Verification items for this drawing (mm, ordinates from the low corner). A direction names the side the tool comes from. Coordinates: 2 decimals unless noted, no trailing zeros. Order: outer loops, then holes, each group sorted by start corner. A loop starts at its lowest first (then second) coordinate and runs counter-clockwise, first axis right, second up. Notation, with made-up numbers: M -26.5,58.25 L 30.5,58.25 A18 cw 30.5,89.25 Z; hole C 48,43.25 d8. An arc over 180 degrees is marked long. Answer as a JSON object with one key per item and string values. Group by question number.
(1) Access from +Z, -Z, +X, -X, +Y, -Y to the whole of each face (thin tool, end or side, straight path). Record for the marked faces 5, 6 and 7.
(2) Material ranges on line 1 (Y direction, x = 15, z = 2.75); line 2 (X direction, y = 10, z = 8.25) (1 decimal); line 3 (X direction, y = 4.75, z = 5.5) (1 decimal), recorded low to high.
(3) Cross-section at D-D (x = 11.5). Enter the section's corners in (y, z).
(4) Cross-section at B-B (z = 6). Enter the section's corners in (x, y) (1 decimal).
(5) Cross-section at C-C (y = 13.5). Enter the section's corners in (x, z), plus the area to 3 significant figures.
(6) Cross-section at A-A (x = 14.75). Enter the section's corners in (y, z).
(7) Mould release check, pull along Y, two halves, no side actions. Record for the marked faces 1, 2, 3 and 4: released by +Y, released by -Y, zero draft, split by the parting line, or undercut.
(8) Gauge pin test, flat ends, axial feed: pin 1 Ø2.5 at (y, z) = (8.5, 3.5) entering from -X; pin 2 Ø4 at (x, z) = (11, 6) entering from -Y; pin 3 Ø2 at (y, z) = (8.5, 2.5) entering from -X. Record the tip position at first contact, or that the pin passes through.
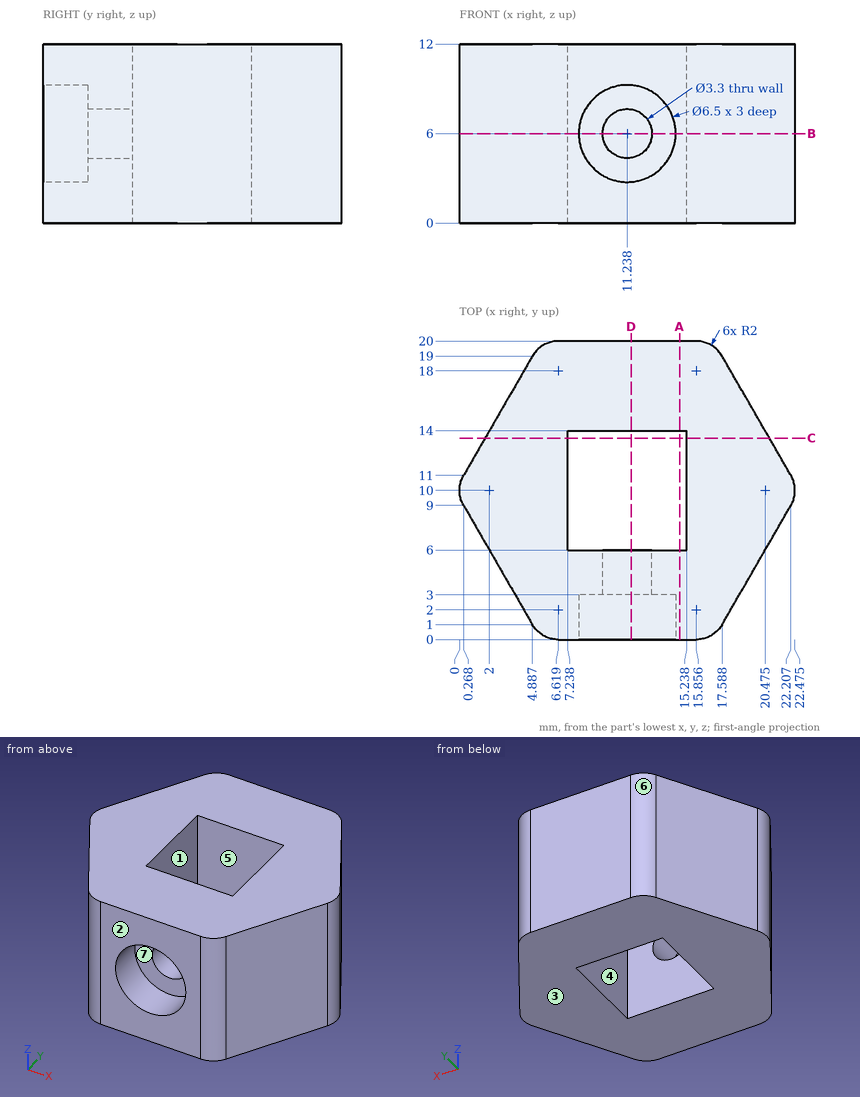
Taken from the geometry:
{
 "1": {"face 5": "+Z, -Z", "face 6": "+Z, -Z, -X, +Y", "face 7": "-Y"},
 "2": {"line 1": "y = 0 to 6, 14 to 20", "line 2": "x = 0 to 7.2, 15.2 to 22.5", "line 3": "x = 2.7 to 9.7, 12.8 to 19.8"},
 "3": {"outline": "M 0,0 L 6,0 L 6,4.37 L 3,4.37 L 3,2.76 L 0,2.76 Z; M 0,9.24 L 3,9.24 L 3,7.63 L 6,7.63 L 6,12 L 0,12 Z; M 14,0 L 20,0 L 20,12 L 14,12 Z"},
 "4": {"outline": "M 0.3,9 L 4.9,1 A2 ccw 6.6,0 L 8,0 L 8,3 L 9.6,3 L 9.6,6 L 7.2,6 L 7.2,14 L 15.2,14 L 15.2,6 L 12.9,6 L 12.9,3 L 14.5,3 L 14.5,0 L 15.9,0 A2 ccw 17.6,1 L 22.2,9 A2 ccw 22.2,11 L 17.6,19 A2 ccw 15.9,20 L 6.6,20 A2 ccw 4.9,19 L 0.3,11 A2 ccw Z"},
 "5": {"outline": "M 1.71,0 L 7.24,0 L 7.24,12 L 1.71,12 Z; M 15.24,0 L 20.76,0 L 20.76,12 L 15.24,12 Z", "area": "133 mm²"},
 "6": {"outline": "M 0,0 L 6,0 L 6,12 L 0,12 Z; M 14,0 L 20,0 L 20,12 L 14,12 Z"},
 "7": {"face 1": "undercut", "face 2": "released by -Y", "face 3": "zero draft", "face 4": "undercut"},
 "8": {"pin 1": "stops at x = 0.02", "pin 2": "stops at y = 3", "pin 3": "stops at x = 0.06"}
}
